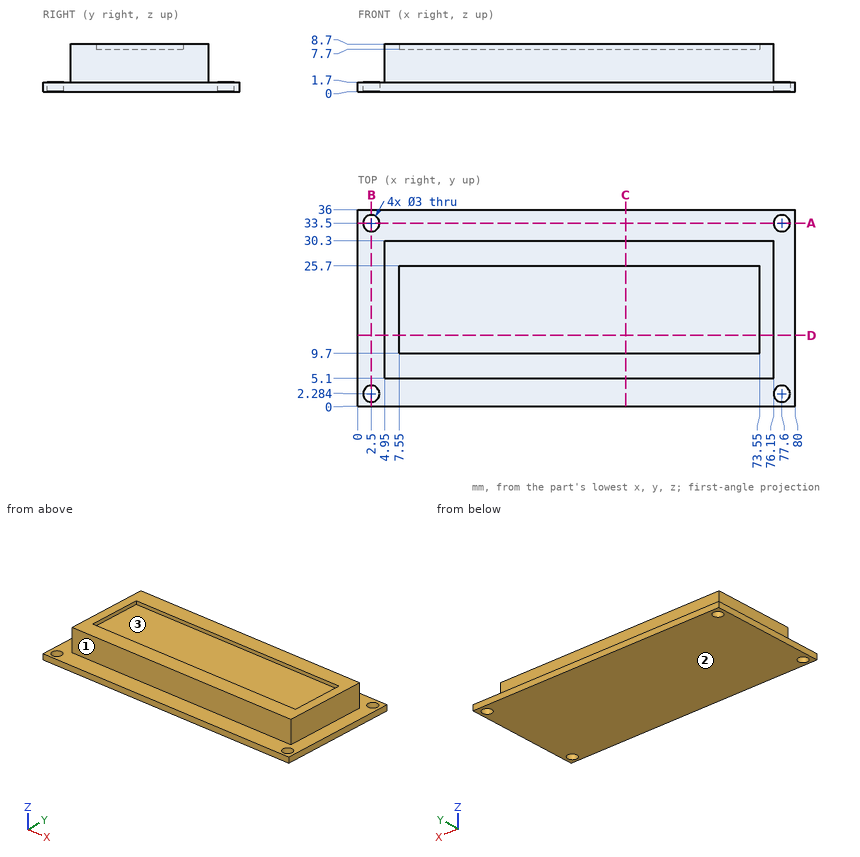
Answer from the drawing. Dimensions are ordinates in mm from the lowest x, y and z of the part. Give positions to 0.01 mm unless a question says otherwise; leave off trailing zeros. Order: outer loops, then holes, each group sorted by start corner. A loop starts at its lowest first (then second) coordinate and runs counter-clockwise, first axis right, second up.
Item 1: For a pull along Y with two mould halves and no side action, classify the marked faces 1, 2 and 3 as pulls with the +Y half, pulls with the -Y half, needs draft (parallel to the pull), parting line crosses it, or undercut.
From the geometry:
face 1: pulls with the -Y half
face 2: needs draft
face 3: undercut
Item 2: The part is cut by section B-B, the plane x = 2.5. Give the vertices of the cut face in (y, z), and give its area (3 significant figures).
From the geometry:
outline: (0, 0) - (0.78, 0) - (0.78, 1.7) - (0, 1.7) - close; (3.78, 0) - (32, 0) - (32, 1.7) - (3.78, 1.7) - close; (35, 0) - (36, 0) - (36, 1.7) - (35, 1.7) - close
area: 51.0 mm2
Item 3: Find the intervals of material crossed by probe 1 along Y at (x, z) = (2.5, 1.1); probe 2 along X at (y, z) = (12, 2); probe 3 along Z at (x, y) = (11, 2), in increasing order.
From the geometry:
probe 1: y = 0 to 0.78, 3.78 to 32, 35 to 36
probe 2: x = 4.95 to 76.15
probe 3: z = 0 to 1.7
Item 4: The part is cut by section D-D, the plane y = 13. Give the vertices of the cut face in (x, z).
From the geometry:
outline: (0, 0) - (80, 0) - (80, 1.7) - (76.15, 1.7) - (76.15, 8.7) - (73.55, 8.7) - (73.55, 7.7) - (7.55, 7.7) - (7.55, 8.7) - (4.95, 8.7) - (4.95, 1.7) - (0, 1.7) - close
Item 5: The part is cut by section C-C, the plane x = 49. Give the vertices of the cut face in (y, z), and give its area (3 significant figures).
From the geometry:
outline: (0, 0) - (36, 0) - (36, 1.7) - (30.3, 1.7) - (30.3, 8.7) - (25.7, 8.7) - (25.7, 7.7) - (9.7, 7.7) - (9.7, 8.7) - (5.1, 8.7) - (5.1, 1.7) - (0, 1.7) - close
area: 222 mm2
Item 6: The part is cut by section A-A, the plane y = 33.5. Give the vertices of the cut face in (x, z).
From the geometry:
outline: (0, 0) - (1, 0) - (1, 1.7) - (0, 1.7) - close; (4, 0) - (76.1, 0) - (76.1, 1.7) - (4, 1.7) - close; (79.1, 0) - (80, 0) - (80, 1.7) - (79.1, 1.7) - close
Item 7: Given pin 1 Ø3 at (x, y) = (8.5, 13.5) entering from -Z; pin 2 Ø3.5 at (y, z) = (11.5, 3.5) entering from +X; pin 3 Ø1.1 at (x, z) = (44.5, 8.5) entering from +Y; pin 4 Ø4 at (y, z) = (24, 7.5) entering from -X, each flat-ended and moving along its own axis, determine where each tip first touches the part or whether it passes through.
From the geometry:
pin 1: stops at z = 0
pin 2: stops at x = 76.15
pin 3: stops at y = 30.3
pin 4: stops at x = 4.95
